Source: CAD feature listing. Evaluate the final solid. Frame: model axes, mm. Coordinates: 2 decimals unless noted, no trailing zeros. Order: outer loops, then holes, each group sorted by start corner. A loop starts at its lowest first (then second) coordinate and runs counter-clockwise, first axis right, second up. Notation, with made-up numbers: (-26.75, 44.25) -> (9.25, 44.25) arc R24 cw to (9.25, 74.25) -> close; hole circle Ø9 at (22, 40). An arc over 180 degrees is marked (long way). Put each result on its own line as item: value.
from build123d import *

# Parameters (mm, degrees)
SKETCH_1_W          = 258
SKETCH_1_H          = 100
EXTRUDE_1_DEPTH     = 4
FILLET_1_R          = 2
SKETCH_2_R          = 1.6
CUT_EXTRUDE_1_DEPTH = 139.408814748
SKETCH_3_R          = 5
CUT_EXTRUDE_2_DEPTH = 139.408814748
FILLET_2_R          = 2
SKETCH_4_R          = 5
CUT_EXTRUDE_3_DEPTH = 139.408814748


with BuildPart() as part:
    # 草图1 → 凸台-拉伸1 (new body)
    with BuildSketch(Plane.XY):
        Rectangle(SKETCH_1_W, SKETCH_1_H)
    extrude(amount=EXTRUDE_1_DEPTH)

    # 圆角1
    fillet_1_edges = [part.edges().sort_by_distance(p)[0] for p in [
        (129, -50, 2),
        (-129, -50, 2),
        (-129, 50, 2),
        (129, 50, 2),
    ]]
    fillet(fillet_1_edges, radius=FILLET_1_R)

    # 草图2 → 切除-拉伸1 (cut, through all)
    with BuildSketch(Plane(origin=(0, 0, 0), x_dir=(-1, 0, 0), z_dir=(0, 0, -1))):
        with Locations((-122, -27)):
            Circle(SKETCH_2_R)
        with Locations((-122, -7)):
            Circle(SKETCH_2_R)
        with Locations((-122, 25)):
            Circle(SKETCH_2_R)
        with Locations((-122, 45)):
            Circle(SKETCH_2_R)
        with Locations((122, -27)):
            Circle(SKETCH_2_R)
        with Locations((122, -7)):
            Circle(SKETCH_2_R)
        with Locations((122, 25)):
            Circle(SKETCH_2_R)
        with Locations((122, 45)):
            Circle(SKETCH_2_R)
    extrude(amount=-CUT_EXTRUDE_1_DEPTH, mode=Mode.SUBTRACT)

    # 草图3 → 切除-拉伸2 (cut, through all)
    with BuildSketch(Plane.XY.offset(4)):
        Polygon((-107, 28.684529573), (-107, -28.684529573), (-62.842544422, 0), align=None)
        Polygon((-24.537386441, 27.5), (-36.084391824, 7.5), (-12.990381057, 7.5), align=None)
        Polygon((-37.527767497, 35), (-89.186600144, 35), (-51.617762103, 10.595413465), align=None)
        Polygon((-51.617762103, -10.595413465), (-89.186600144, -35), (-37.527767497, -35), align=None)
        Polygon((-12.990381057, -7.5), (-36.084391824, -7.5), (-24.537386441, -27.5), align=None)
        Polygon((0, -15), (-11.547005384, -35), (11.547005384, -35), align=None)
        Polygon((-11.547005384, 35), (0, 15), (11.547005384, 35), align=None)
        Polygon((36.084391824, -7.5), (12.990381057, -7.5), (24.537386441, -27.5), align=None)
        Polygon((89.186600144, 35), (37.527767497, 35), (51.617762103, 10.595413465), align=None)
        Polygon((107, 28.684529573), (62.842544422, 0), (107, -28.684529573), align=None)
        Polygon((89.186600144, -35), (51.617762103, -10.595413465), (37.527767497, -35), align=None)
        Polygon((24.537386441, 27.5), (12.990381057, 7.5), (36.084391824, 7.5), align=None)
        with Locations((-49.074772881, 0)):
            Circle(SKETCH_3_R)
        with Locations((49.074772881, 0)):
            Circle(SKETCH_3_R)
    extrude(amount=-CUT_EXTRUDE_2_DEPTH, mode=Mode.SUBTRACT)

    # 圆角2
    fillet_2_edges = [part.edges().sort_by_distance(p)[0] for p in [
        (-24.537386441, 27.5, 2),
        (-12.990381057, 7.5, 2),
        (-36.084391824, 7.5, 2),
        (-37.527767497, 35, 2),
        (-51.617762103, 10.595413465, 2),
        (-89.186600144, 35, 2),
        (-89.186600144, -35, 2),
        (-51.617762103, -10.595413465, 2),
        (-37.527767497, -35, 2),
        (-12.990381057, -7.5, 2),
        (-24.537386441, -27.5, 2),
        (-36.084391824, -7.5, 2),
        (-11.547005384, -35, 2),
        (0, -15, 2),
        (11.547005384, -35, 2),
        (11.547005384, 35, 2),
        (0, 15, 2),
        (-11.547005384, 35, 2),
        (24.537386441, -27.5, 2),
        (12.990381057, -7.5, 2),
        (36.084391824, -7.5, 2),
        (37.527767497, 35, 2),
        (89.186600144, 35, 2),
        (51.617762103, 10.595413465, 2),
        (36.084391824, 7.5, 2),
        (12.990381057, 7.5, 2),
        (24.537386441, 27.5, 2),
        (107, -28.684529573, 2),
        (62.842544422, 0, 2),
        (107, 28.684529573, 2),
        (37.527767497, -35, 2),
        (51.617762103, -10.595413465, 2),
        (89.186600144, -35, 2),
        (-62.842544422, 0, 2),
        (-107, -28.684529573, 2),
        (-107, 28.684529573, 2),
    ]]
    fillet(fillet_2_edges, radius=FILLET_2_R)

    # 草图4 → 切除-拉伸3 (cut, through all)
    with BuildSketch(Plane.XY.offset(4)):
        Circle(SKETCH_4_R)
    extrude(amount=-CUT_EXTRUDE_3_DEPTH, mode=Mode.SUBTRACT)


solid = part.part
1. First-contact query: pin 1 (3 mm diameter, centred on x = -122, y = -7, fed in from +Z); pin 2 (3.5 mm diameter, centred on x = -122, y = -27, fed in from +Z). Flat tips, straight axial feed; report the tip coordinate or a pass-through.
Numbers:
pin 1: passes through
pin 2: stops at z = 4
2. Cut plane B-B on z = 0.75. Count the separate pieces of the cut face and the enclosed holes in it, plus the area to 3 significant figures.
Numbers:
separate pieces: 1
enclosed holes: 23
area: 19,200 mm2
3. Cut plane A-A on x = -48. Output: boundary loops of the cut face in (y, z).
Numbers:
outline: (-50, 0) -> (-35, 0) -> (-35, 4) -> (-50, 4) -> close; (-16.86, 0) -> (-4.88, 0) -> (-4.88, 4) -> (-16.86, 4) -> close; (4.88, 0) -> (16.86, 0) -> (16.86, 4) -> (4.88, 4) -> close; (35, 0) -> (50, 0) -> (50, 4) -> (35, 4) -> close
4. Cut plane C-C on x = 79.5. Output: boundary loops of the cut face in (y, z), plus the area to 3 significant figures.
Numbers:
outline: (-50, 0) -> (-35, 0) -> (-35, 4) -> (-50, 4) -> close; (-28.71, 0) -> (-10.82, 0) -> (-10.82, 4) -> (-28.71, 4) -> close; (10.82, 0) -> (28.71, 0) -> (28.71, 4) -> (10.82, 4) -> close; (35, 0) -> (50, 0) -> (50, 4) -> (35, 4) -> close
area: 263 mm2
5. Ray query, line 1 along Y through (x, z) = (63, 1.6); line 2 along Y through (x, z) = (-122, 1.7); line 3 along X through (y, z) = (-2, 3.45). Return the intervals inside material, ascending.
Numbers:
line 1: y = -50 to -35, -17.99 to 17.99, 35 to 50
line 2: y = -50 to -28.6, -25.4 to -8.6, -5.4 to 23.4, 26.6 to 43.4, 46.6 to 50
line 3: x = -129 to -107, -65.92 to -53.66, -44.49 to -4.58, 4.58 to 44.49, 53.66 to 65.92, 107 to 129
